Geometry: final body of the model. Coordinates: model frame, mm. A direction names the side the tool comes from. Coordinates: 2 decimals unless noted, no trailing zeros. Loops run counter-clockwise (first coordinate to the right, second up) from the corner with the lowest first, then second, coordinate; pieces in that order, holes last. Notation, with made-up numbers: (-31.5, 89) - (14.5, 89) arc R17 ccw to (14.5, 99) - close; hole circle Ø9 at (30.25, 61.5). An arc over 180 degrees is marked (long way). Put each result on its own line as item: value. Start each with the question number.
1) Section A-A on z = 27.25. Output: boundary loops of the cut face in (x, y), and give its area (3 significant figures).
2) Contact query for flat-ended pins moving along their axis: pin 1 Ø5 at (y, z) = (-25, 24) entering from +X; pin 2 Ø4 at (y, z) = (-115.5, 9.5) entering from -X; pin 3 Ø8 at (x, z) = (-23.5, 12) entering from +Y. Output: stop coordinate, or through.
3) Section B-B on y = 0. Output: boundary loops of the cut face in (x, z), and give its area (3 significant figures).
4) Section C-C on x = 6. Output: boundary loops of the cut face in (y, z), and give its area (3 significant figures).
5) Section D-D on y = -176. Output: boundary loops of the cut face in (x, z).
6) Material intervals for line 1 along Y through (x, z) = (0, 17.75); line 2 along X through (y, z) = (-100, 17); line 3 along X through (y, z) = (-105.5, 12), sorted ascending. Write a range as from..to.
7) Draft query along X for faces 1 (the cylindrical face through (14.394, -137.016, 14.79)), 2 (the cylindrical face through (0, 28, 15)), 3 (the cylindrical face through (-44.73, -197.81, 14.79)), 4 (the flat face through (-1, -89, 30)). Return one class per face: +X half, -X half, draft (parallel to the pull), parting line (faces both ways), or undercut.
8) Reachability of faces 5 (the flat face through (-42.96, -32.19, 14.79)), 6 (the cylindrical face through (-46.902, -207.572, 14.79)) from +Z, -Z, +X, -X, +Y, -Y: full face, straight path, thin tool, end or side. Return the list, or none.
```python
from build123d import *

# Parameters (mm, degrees)
SKETCH2_R           = 17
BOSS_EXTRUDE1_DEPTH = 30
SKETCH2_4_R         = 18
SKETCH2_4_R_2       = 8
BOSS_EXTRUDE2_DEPTH = 30
BOSS_EXTRUDE3_DEPTH = 5


with BuildPart() as part:
    # Sketch2 → Boss-Extrude1 (new body)
    with BuildSketch(Plane.XY):
        with BuildLine():
            Line((60.387064012, -75.95), (26.012889113, 10.36))
            ThreePointArc((26.012889113, 10.36), (0, 28), (-26.012889113, 10.36))
            Line((-26.012889113, 10.36), (-60.387064012, -75.95))
            ThreePointArc((-60.387064012, -75.95), (-63.836349993, -87.755800573), (-65, -100))
            Line((-65, -100), (-64.745963704, -105.741096069))
            ThreePointArc((-64.745963704, -105.741096069), (-43.885241002, -147.948781238), (0, -165))
            ThreePointArc((0, -165), (53.797072411, -136.481159521), (60.387064012, -75.95))
        make_face()
        with BuildLine():
            ThreePointArc((-37.165332046, -136.369466506), (0.28138508, -48.000761328), (36.769552622, -136.769552622))
            ThreePointArc((36.769552622, -136.769552622), (14.142135624, -136.769552622), (14.142135624, -114.142135624))
            ThreePointArc((14.142135624, -114.142135624), (0.108225031, -80.000292819), (-14.294358479, -113.988256349))
            ThreePointArc((-14.294358479, -113.988256349), (-14.539240183, -136.614348211), (-37.165332046, -136.369466506))
        make_face(mode=Mode.SUBTRACT)
        Circle(SKETCH2_R, mode=Mode.SUBTRACT)
    extrude(amount=BOSS_EXTRUDE1_DEPTH)



with BuildPart() as body_2:
    # Sketch2<4> → Boss-Extrude2 (new body)
    with BuildSketch(Plane.XY):
        with Locations((-43, -190)):
            Circle(SKETCH2_4_R)
        with Locations((-43, -190)):
            Circle(SKETCH2_4_R_2, mode=Mode.SUBTRACT)
    extrude(amount=BOSS_EXTRUDE2_DEPTH)


with BuildPart() as part_1:
    add(part.part)

    add(body_2.part)  # Boss-Extrude3 merges body 2
    # Sketch3 → Boss-Extrude3 (add)
    with BuildSketch(Plane.XY):
        with BuildLine():
            ThreePointArc((2.030385563, -164.968280987), (-43.130914594, -148.62843002), (-64.745963704, -105.741096069))
            Line((-64.745963704, -105.741096069), (-61, -190))
            ThreePointArc((-61, -190), (-43, -172), (-25, -190))
            ThreePointArc((-25, -190), (-25.009294588, -190.578375974), (-25.037168752, -191.15615464))
            ThreePointArc((-25.037168752, -191.15615464), (-16.564278272, -172.831330157), (2.030385563, -164.968280987))
        make_face()
    extrude(amount=BOSS_EXTRUDE3_DEPTH)


solid = part_1.part
```
Answer block:
1. outline: (-65, -100) - (-64.75, -105.74) arc R65 ccw (long way) to (60.39, -75.95) - (26.01, 10.36) arc R28 ccw to (-26.01, 10.36) - (-60.39, -75.95) arc R65 ccw to start; circle Ø36 at (-43, -190); hole circle Ø16 at (-43, -190); hole (-37.17, -136.37) arc R16 ccw to (-14.29, -113.99) arc R20 cw (long way) to (14.14, -114.14) arc R16 ccw to (36.77, -136.77) arc R52 ccw (long way) to start; hole circle Ø34 at (0, 0)
1. area: 11,500 mm²
2. pin 1: stops at x = 41.09
2. pin 2: stops at x = -63.58
2. pin 3: stops at y = 20.09
3. outline: (-30.14, 0) - (-17, 0) - (-17, 30) - (-30.14, 30) - close; (17, 0) - (30.14, 0) - (30.14, 30) - (17, 30) - close
3. area: 788 mm²
4. outline: (-164.72, 0) - (-80.92, 0) - (-80.92, 30) - (-164.72, 30) - close; (-48.35, 0) - (-15.91, 0) - (-15.91, 30) - (-48.35, 30) - close; (15.91, 0) - (27.35, 0) - (27.35, 30) - (15.91, 30) - close
4. area: 3,830 mm²
5. outline: (-61.62, 0) - (-19.38, 0) - (-19.38, 5) - (-31.69, 5) - (-31.69, 30) - (-54.31, 30) - (-54.31, 5) - (-61.62, 5) - close
6. line 1: y = -165..-80, -48..-17, 17..28
6. line 2: x = -65..-52, -20..20, 52..65
6. line 3: x = -64.76..-51.71, -19.23..19.23, 51.71..64.77
7. face 1: undercut
7. face 2: parting line
7. face 3: undercut
7. face 4: draft
8. face 5: +Z, -Z, -X, +Y
8. face 6: +Z
